from build123d import *

# Parameters (mm, degrees)
SKETCH_1_W          = 272
SKETCH_1_H          = 121
EXTRUDE_1_DEPTH     = 2
SKETCH_2_R          = 2.1
CUT_EXTRUDE_1_DEPTH = 149.863192227
FILLET_1_R          = 2
SKETCH_3_R          = 2.1
SKETCH_3_R_2        = 2.06
SKETCH_3_R_3        = 48
CUT_EXTRUDE_2_DEPTH = 149.863192227


with BuildPart() as part:
    # 草图1 → 凸台-拉伸1 (new body)
    with BuildSketch(Plane(origin=(0, 0, 0), x_dir=(1, 0, 0), z_dir=(0, 1, 0))):
        Rectangle(SKETCH_1_W, SKETCH_1_H)
    extrude(amount=EXTRUDE_1_DEPTH)

    # 草图2 → 切除-拉伸1 (cut, through all)
    with BuildSketch(Plane(origin=(0, 2, 0), x_dir=(1, 0, 0), z_dir=(0, 1, 0))):
        with Locations(Location((121, 50.5, 0), (0, 0, 270))):
            Circle(SKETCH_2_R)
        with Locations(Location((121, 32.5, 0), (0, 0, 270))):
            Circle(SKETCH_2_R)
        with Locations(Location((121, -32.5, 0), (0, 0, 90))):
            Circle(SKETCH_2_R)
        with Locations(Location((121, -50.5, 0), (0, 0, 90))):
            Circle(SKETCH_2_R)
        with Locations(Location((-121, -50.5, 0), (0, 0, 270))):
            Circle(SKETCH_2_R)
        with Locations(Location((-121, -32.5, 0), (0, 0, 270))):
            Circle(SKETCH_2_R)
        with Locations(Location((-121, 32.5, 0), (0, 0, 90))):
            Circle(SKETCH_2_R)
        with Locations(Location((-121, 50.5, 0), (0, 0, 90))):
            Circle(SKETCH_2_R)
    extrude(amount=-CUT_EXTRUDE_1_DEPTH, mode=Mode.SUBTRACT)

    # 圆角1
    fillet_1_edges = [part.edges().sort_by_distance(p)[0] for p in [
        (136, 1, 60.5),
        (-136, 1, 60.5),
        (-136, 1, -60.5),
        (136, 1, -60.5),
    ]]
    fillet(fillet_1_edges, radius=FILLET_1_R)

    # 草图3 → 切除-拉伸2 (cut, through all)
    with BuildSketch(Plane.XZ):
        with Locations(Location((-13.75, -38.25, 0), (0, 0, 270))):
            Circle(SKETCH_3_R)
        with Locations(Location((-13.75, 38.25, 0), (0, 0, 270))):
            Circle(SKETCH_3_R_2)
        with Locations(Location((-90.25, 38.25, 0), (0, 0, 270))):
            Circle(SKETCH_3_R)
        with Locations(Location((-90.25, -38.25, 0), (0, 0, 270))):
            Circle(SKETCH_3_R)
        with Locations(Location((-52, 0, 0), (0, 0, 270))):
            Circle(SKETCH_3_R_3)
    extrude(amount=-CUT_EXTRUDE_2_DEPTH, mode=Mode.SUBTRACT)


solid = part.part
Model file for the job. Use its own axes, mm. Round coordinates to 2 decimals unless told otherwise and drop trailing zeros. Loops run counter-clockwise (first coordinate to the right, second up) from the corner with the lowest first, then second, coordinate; pieces in that order, holes last. Notation, with made-up numbers: (9.5, -9.75) - (19.5, -9.75) arc R12 cw to (19.5, -1.75) - close; hole circle Ø2 at (64, 39). An arc over 180 degrees is marked (long way). Write each question's results on one line, items separated by ' | '.
(1) Saw through at A-A, the plane x = -52. List the corners of the cut face in (y, z), then the cut area to 3 significant figures.
Answer below:
outline: (0, -60.5) - (2, -60.5) - (2, -48) - (0, -48) - close; (0, 48) - (2, 48) - (2, 60.5) - (0, 60.5) - close | area: 50.0 mm^2
(2) Saw through at C-C, the plane y = 0.7. Count the separate pieces of the cut face and the enclosed holes in it, then the cut area to 3 significant figures.
Answer below:
separate pieces: 1 | enclosed holes: 13 | area: 25,500 mm^2
(3) Wall check: L1, parallel to X at y = 1.3, z = -50.5; L2, parallel to X at y = 0.65, z = -49; L3, parallel to X at y = 1.55, z = 32.5. Give the ranges that are in metal, low to high.
Answer below:
L1: x = -136 to -123.1, -118.9 to 118.9, 123.1 to 136 | L2: x = -136 to -122.47, -119.53 to 119.53, 122.47 to 136 | L3: x = -136 to -123.1, -118.9 to -87.32, -16.68 to 118.9, 123.1 to 136
(4) Saw through at B-B, the plane z = 0. List the corners of the cut face in (x, y), then the cut area to 3 significant figures.
Answer below:
outline: (-136, 0) - (-100, 0) - (-100, 2) - (-136, 2) - close; (-4, 0) - (136, 0) - (136, 2) - (-4, 2) - close | area: 352 mm^2
(5) Mould opens along Z. For faces 1 (the flat face through (-2, 2, -1)), 2 (the cylindrical face through (-94.584, 0.986, -22.149)) say: released by +Z, released by -Z, zero draft, split by the parting line, or undercut.
Answer below:
face 1: zero draft | face 2: undercut
